Model file for the job. Use its own axes, mm. A direction names the side the tool comes from. Round coordinates to 2 decimals unless told otherwise and drop trailing zeros. Order: outer loops, then holes, each group sorted by start corner. A loop starts at its lowest first (then second) coordinate and runs counter-clockwise, first axis right, second up. Notation, with made-up numbers: M 20,2.25 L 52,2.25 A15 ccw 52,25.25 Z; hole C 59.25,77 d3. An arc over 180 degrees is marked long. Return JSON: item names as keys, results as strings. Group by question number.
Item 1: Pin check, flat tips, straight feed: pin 1 Ø5.5 at (y, z) = (0, 0) entering from +X; pin 2 Ø1 at (x, z) = (1, 3) entering from -Y; pin 3 Ø1.5 at (x, z) = (2, -4) entering from -Y; pin 4 Ø0.9 at (x, z) = (1, 28) entering from -Y. Stop position of each tip, or through.
Item 2: Slice it at A-A on z = 0. Write the cut outline in (x, y), then the cut area to 3 significant figures.
Item 3: Pull direction Z, two halves, no side cores. Call faces 4 (the face through (1.479, -23.635, -46.076)), 5 (the face through (0, -7, 4)), 6 (the face through (1, -8, 0)): pulls with the +Z half, pulls with the -Z half, needs draft (parallel to the pull), parting line crosses it, or undercut.
Item 4: Which spindle directions (+Z, -Z, +X, -X, +Y, -Y) get a long thin tool onto all of the face, cutting with end or side? Do faces 1 (the face through (1, -25, 42)), 2 (the face through (1, -25, -42)), 3 (the face through (1.479, -19.2, -29.127)). Say none if no direction does.
Item 5: Slice it at D-D on z = 39. Write the cut outline in (x, y), then the cut area to 3 significant figures.
Item 6: Slice it at B-B on x = 0.65. Write the cut outline in (y, z).
Item 7: Probe line 1 along Z through (x, y) = (0.5, -23.5); line 2 along Y through (x, z) = (0.75, 0); line 3 along Z through (x, y) = (2.7, -24). List the from-to ranges inside material, lowest first.
Item 8: Slice it at C-C on y = -15.5. Write the cut outline in (x, z).
from build123d import *

# Parameters (mm, degrees)
SKETCH1_R           = 3.45
SKETCH1_R_2         = 1.1
BOSS_EXTRUDE1_DEPTH = 3


with BuildPart() as part:
    # Sketch1 → Boss-Extrude1 (new body)
    with BuildSketch(Plane(origin=(0, 0, 0), x_dir=(0, 0, -1), z_dir=(1, 0, 0))):
        with BuildLine():
            Line((-4.875399709, 6.962792376), (-45.326961199, -21.361695911))
            ThreePointArc((-45.326961199, -21.361695911), (-46.087242228, -23.601411599), (-44.179808327, -25))
            Line((-44.179808327, -25), (-40.062317158, -25))
            Line((-40.062317158, -25), (-29.999489725, -17.953932376))
            Line((-29.999489725, -17.953932376), (-28.278760416, -20.411388509))
            Line((-28.278760416, -20.411388509), (-34.831976771, -25))
            Line((-34.831976771, -25), (-22.712020043, -25))
            ThreePointArc((-22.712020043, -25), (0, -8), (22.324675322, -25.505562722))
            Line((22.324675322, -25.505562722), (34.831976771, -25))
            Line((34.831976771, -25), (28.278760416, -20.411388509))
            Line((28.278760416, -20.411388509), (29.999489725, -17.953932376))
            Line((29.999489725, -17.953932376), (40.062317158, -25))
            Line((40.062317158, -25), (44.179808327, -25))
            ThreePointArc((44.179808327, -25), (46.087242228, -23.601411599), (45.326961199, -21.361695911))
            Line((45.326961199, -21.361695911), (4.875399709, 6.962792376))
            ThreePointArc((4.875399709, 6.962792376), (0, 8.5), (-4.875399709, 6.962792376))
        make_face()
        Circle(SKETCH1_R, mode=Mode.SUBTRACT)
        with Locations((-13.491798398, -5.174347881)):
            Circle(SKETCH1_R_2, mode=Mode.SUBTRACT)
    extrude(amount=BOSS_EXTRUDE1_DEPTH)


solid = part.part
Output values:
{
 "1": {"pin 1": "through", "pin 2": "y = -8.22", "pin 3": "y = -8.54", "pin 4": "y = -25"},
 "2": {"outline": "M 0,-8 L 3,-8 L 3,-3.45 L 0,-3.45 Z; M 0,3.45 L 3,3.45 L 3,8.5 L 0,8.5 Z", "area": "28.8 mm²"},
 "3": {"face 4": "pulls with the -Z half", "face 5": "needs draft", "face 6": "undercut"},
 "4": {"face 1": "+Z, +X, -X, -Y", "face 2": "-Z, +X, -X, -Y", "face 3": "+X, -X"},
 "5": {"outline": "M 0,-24.26 L 3,-24.26 L 3,-16.93 L 0,-16.93 Z", "area": "22.0 mm²"},
 "6": {"outline": "M -25.51,-22.32 L -25,-34.83 L -20.41,-28.28 L -17.95,-30 L -25,-40.06 L -25,-44.18 A2 ccw -21.36,-45.33 L 6.96,-4.88 A8.5 ccw 6.96,4.88 L -21.36,45.33 A2 ccw -25,44.18 L -25,40.06 L -17.95,30 L -20.41,28.28 L -25,34.83 L -25,22.71 A23.32 cw Z; hole C -5.17,13.49 d2.2; hole C 0,0 d6.9"},
 "7": {"line 1": "-46.12 to -37.92, -32.69 to -21.71, 22.23 to 32.69, 37.92 to 46.12", "line 2": "-8 to -3.45, 3.45 to 8.5", "line 3": "-45.91 to -38.63, -33.4 to -21.88, 22.41 to 33.4, 38.63 to 45.91"},
 "8": {"outline": "M 0,-36.96 L 3,-36.96 L 3,-16.87 L 0,-16.87 Z; M 0,17.4 L 3,17.4 L 3,36.96 L 0,36.96 Z"}
}
